```python
from build123d import *

# Parameters (mm, degrees)
SKETCH2_W           = 38.1
SKETCH2_H           = 50.8
BOSS_EXTRUDE1_DEPTH = 1.5875
SKETCH3_W           = 1.5875
SKETCH3_H           = 50.8
BOSS_EXTRUDE2_DEPTH = 38.1
CUT_EXTRUDE1_REACH  = 62.596
SKETCH4_R           = 1.778
SKETCH4_R_2         = 1.27


with BuildPart() as part:
    # Sketch2 → Boss-Extrude1 (new body)
    with BuildSketch(Plane(origin=(0, 0, 0), x_dir=(0, 0, -1), z_dir=(1, 0, 0))):
        Rectangle(SKETCH2_W, SKETCH2_H)
    extrude(amount=BOSS_EXTRUDE1_DEPTH)

    # Sketch3 → Boss-Extrude2 (add)
    with BuildSketch(Plane(origin=(1.5875, 0, 0), x_dir=(0, 0, -1), z_dir=(1, 0, 0))):
        with Locations((-18.25625, 0)):
            Rectangle(SKETCH3_W, SKETCH3_H)
    extrude(amount=BOSS_EXTRUDE2_DEPTH)

    # Sketch4 → Cut-Extrude1 (cut, up to next)
    with BuildSketch(Plane.XY.offset(19.05), mode=Mode.PRIVATE) as cut_extrude1_sk1:
        with Locations((21.9075, 0)):
            Circle(SKETCH4_R)
    cut_extrude1_tool1 = extrude(cut_extrude1_sk1.sketch, amount=-CUT_EXTRUDE1_REACH, mode=Mode.PRIVATE) & part.part
    # Sketch4 → Cut-Extrude1 (cut, up to next)
    with BuildSketch(Plane.XY.offset(19.05), mode=Mode.PRIVATE) as cut_extrude1_sk2:
        with Locations((21.9075, 8.763)):
            Circle(SKETCH4_R_2)
    cut_extrude1_tool2 = extrude(cut_extrude1_sk2.sketch, amount=-CUT_EXTRUDE1_REACH, mode=Mode.PRIVATE) & part.part
    # Sketch4 → Cut-Extrude1 (cut, up to next)
    with BuildSketch(Plane.XY.offset(19.05), mode=Mode.PRIVATE) as cut_extrude1_sk3:
        with Locations((21.9075, -8.763)):
            Circle(SKETCH4_R_2)
    cut_extrude1_tool3 = extrude(cut_extrude1_sk3.sketch, amount=-CUT_EXTRUDE1_REACH, mode=Mode.PRIVATE) & part.part
    add(cut_extrude1_tool1.solids().sort_by_distance((21.9075, 0, 19.05))[0], mode=Mode.SUBTRACT)
    add(cut_extrude1_tool2.solids().sort_by_distance((21.9075, 8.763, 19.05))[0], mode=Mode.SUBTRACT)
    add(cut_extrude1_tool3.solids().sort_by_distance((21.9075, -8.763, 19.05))[0], mode=Mode.SUBTRACT)


solid = part.part
```
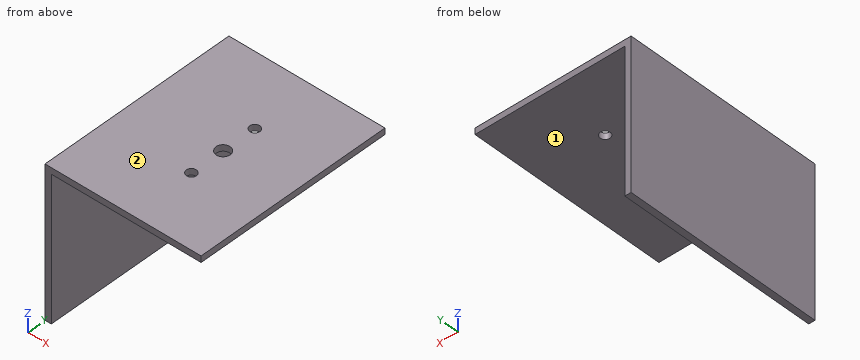
Geometry: final body of the model. Coordinates: model frame, mm. Face numbers are marked on the shaded views. A direction names the side the tool comes from. Coordinates: 2 decimals unless noted, no trailing zeros. Order: outer loops, then holes, each group sorted by start corner. A loop starts at its lowest first (then second) coordinate and runs counter-clockwise, first axis right, second up. Notation, with made-up numbers: (70.25, -35) -> (115.25, -35) arc R22 cw to (115.25, -28) -> close; hole circle Ø10 at (-6.5, 35.25). An arc over 180 degrees is marked (long way). Use CSV: the item, a comma, the result in double quotes.
1) Pin query (flat end, axial travel): pin 1 Ø12 at (y, z) = (1, 2.5) entering from +X; pin 2 Ø1.5 at (x, y) = (21.91, -8.76) entering from -Z. Return the tip coordinate at first contact, or that it passes through.
Findings:
pin 1,"stops at x = 1.59"
pin 2,"passes through"
2) Line query: line 1 (Z direction, x = 9.5, y = -20); line 2 (X direction, y = -6, z = 8). Output: solid intervals per line, ascending.
Findings:
line 1,"z = 17.46 to 19.05"
line 2,"x = 0 to 1.59"
3) Section C-C on y = 21. Output: boundary loops of the cut face in (x, z), then the cut area to 3 significant figures.
Findings:
outline,"(0, -19.05) -> (1.59, -19.05) -> (1.59, 17.46) -> (39.69, 17.46) -> (39.69, 19.05) -> (0, 19.05) -> close"
area,"121 mm^2"
4) Section B-B on x = 16.5. Output: boundary loops of the cut face in (y, z), then the cut area to 3 significant figures.
Findings:
outline,"(-25.4, 17.46) -> (25.4, 17.46) -> (25.4, 19.05) -> (-25.4, 19.05) -> close"
area,"80.6 mm^2"
5) Section A-A on y = 0. Output: boundary loops of the cut face in (x, z).
Findings:
outline,"(0, -19.05) -> (1.59, -19.05) -> (1.59, 17.46) -> (20.13, 17.46) -> (20.13, 19.05) -> (0, 19.05) -> close; (23.69, 17.46) -> (39.69, 17.46) -> (39.69, 19.05) -> (23.69, 19.05) -> close"
6) Section D-D on z = -12.5. Output: boundary loops of the cut face in (x, y), then the cut area to 3 significant figures.
Findings:
outline,"(0, -25.4) -> (1.59, -25.4) -> (1.59, 25.4) -> (0, 25.4) -> close"
area,"80.6 mm^2"
7) Access query for the marked faces 1 and 2. Directions: +Z, -Z, +X, -X, +Y, -Y. A direction counts if a zero-diameter tool reaches every point of the face in a straight line with its end or side. Return the directions, or none.
Findings:
face 1,"-Z, +X, +Y, -Y"
face 2,"+Z, +X, -X, +Y, -Y"
